from build123d import *

# Parameters (mm, degrees)
BOSS_EXTRUDE1_DEPTH     = 10
BOSS_EXTRUDE2_START     = 2.8
BOSS_EXTRUDE2_DEPTH     = 4.4
BOSS_EXTRUDE3_DEPTH     = 45
CUT_EXTRUDE1_DEPTH      = 103.347447452
CUT_EXTRUDE1_DEPTH_BACK = 103.347447452
CUT_EXTRUDE2_START      = -35
CUT_EXTRUDE2_DEPTH      = 35
SKETCH7_R               = 2.625
CUT_EXTRUDE5_DEPTH      = 43.5


with BuildPart() as part:
    # Sketch1 → Boss-Extrude1 (new body)
    with BuildSketch(Plane(origin=(0, 0, 0), x_dir=(1, 0, 0), z_dir=(0, 1, 0))):
        with BuildLine():
            Line((-40.2, -57.876303889), (-40.2, 0))
            ThreePointArc((-40.2, 0), (-36.256585609, 17.363755354), (-25.2, 31.320919527))
            ThreePointArc((-25.2, 31.320919527), (0, 40.2), (25.2, 31.320919527))
            ThreePointArc((25.2, 31.320919527), (36.256585609, 17.363755354), (40.2, 0))
            Line((40.2, 0), (40.2, -57.876303889))
            ThreePointArc((40.2, -57.876303889), (41.890773052, -60.2417112), (44.676121397, -59.40762496))
            ThreePointArc((44.676121397, -59.40762496), (50.25367708, -51.409776352), (55, -42.892316139))
            Line((55, -42.892316139), (55, 0))
            ThreePointArc((55, 0), (0, 55), (-55, 0))
            Line((-55, 0), (-55, -42.892316139))
            ThreePointArc((-55, -42.892316139), (-50.25367708, -51.409776352), (-44.676121397, -59.40762496))
            ThreePointArc((-44.676121397, -59.40762496), (-41.890773052, -60.2417112), (-40.2, -57.876303889))
        make_face()
    extrude(amount=BOSS_EXTRUDE1_DEPTH)

    # Sketch1<5> → Boss-Extrude2 (add)
    with BuildSketch(Plane(origin=(0, 0, 0), x_dir=(1, 0, 0), z_dir=(0, 1, 0)).offset(BOSS_EXTRUDE2_START)):
        with BuildLine():
            ThreePointArc((-25.2, 31.320919527), (-36.256585609, 17.363755354), (-40.2, 0))
            Line((-40.2, 0), (-40.2, -57.876303889))
            Line((-40.2, -57.876303889), (-29.879111138, -45.576347508))
            ThreePointArc((-29.879111138, -45.576347508), (-26.406147584, -39.560998181), (-25.2, -32.720595315))
            Line((-25.2, -32.720595315), (-25.2, 31.320919527))
        make_face()
        with BuildLine():
            ThreePointArc((40.2, 0), (36.256585609, 17.363755354), (25.2, 31.320919527))
            Line((25.2, 31.320919527), (25.2, -32.720595315))
            ThreePointArc((25.2, -32.720595315), (26.406147584, -39.560998181), (29.879111138, -45.576347508))
            Line((29.879111138, -45.576347508), (40.2, -57.876303889))
            Line((40.2, -57.876303889), (40.2, 0))
        make_face()
    extrude(amount=BOSS_EXTRUDE2_DEPTH)

    # Sketch1<6> → Boss-Extrude3 (add)
    with BuildSketch(Plane(origin=(0, 0, 0), x_dir=(1, 0, 0), z_dir=(0, 1, 0))):
        with BuildLine():
            ThreePointArc((-65, 0), (-62.466921066, -22.021300959), (-55, -42.892316139))
            Line((-55, -42.892316139), (-55, 0))
            ThreePointArc((-55, 0), (0, 55), (55, 0))
            Line((55, 0), (55, -42.892316139))
            ThreePointArc((55, -42.892316139), (62.466921066, -22.021300959), (65, 0))
            ThreePointArc((65, 0), (0, 65), (-65, 0))
        make_face()
    extrude(amount=BOSS_EXTRUDE3_DEPTH)

    # Sketch2 → Cut-Extrude1 (cut, two sides: drawn at the far end of the back side and taken through both)
    with BuildSketch(Plane(origin=(0, 0, 0), x_dir=(0, 0, -1), z_dir=(1, 0, 0)).offset(-CUT_EXTRUDE1_DEPTH_BACK)):
        with BuildLine():
            Line((-42.892316139, 10), (-42.892316139, 45))
            Line((-42.892316139, 45), (17.107683861, 45))
            ThreePointArc((17.107683861, 45), (-17.623426113, 35.61047424), (-42.892316139, 10))
        make_face()
    extrude(amount=CUT_EXTRUDE1_DEPTH + CUT_EXTRUDE1_DEPTH_BACK, mode=Mode.SUBTRACT)

    # Sketch3 → Cut-Extrude2 (cut)
    with BuildSketch(Plane(origin=(0, 45, 0), x_dir=(1, 0, 0), z_dir=(0, 1, 0)).offset(CUT_EXTRUDE2_START)):
        with BuildLine():
            Line((-34.164958741, 55.296976357), (-27.5, 47.631397208))
            ThreePointArc((-27.5, 47.631397208), (-36.087479082, 41.505347288), (-43.347496237, 33.852541558))
            ThreePointArc((-43.347496237, 33.852541558), (-47.000937608, 28.564170983), (-50.012454978, 22.885679957))
            Line((-50.012454978, 22.885679957), (-50.012454978, 41.518120707))
            ThreePointArc((-50.012454978, 41.518120707), (-42.648838916, 49.051774067), (-34.164958741, 55.296976357))
        make_face()
        with BuildLine():
            Line((64.971065648, 1.93923401), (55, 0))
            ThreePointArc((55, 0), (53.988424685, 10.5), (50.990909091, 20.613762153))
            ThreePointArc((50.990909091, 20.613762153), (48.237766513, 26.421920479), (44.825807714, 31.869216538))
            Line((44.825807714, 31.869216538), (60.961974739, 22.552996163))
            ThreePointArc((60.961974739, 22.552996163), (63.804501901, 12.409090909), (64.971065648, 1.93923401))
        make_face()
    extrude(amount=CUT_EXTRUDE2_DEPTH, mode=Mode.SUBTRACT)

    # Sketch7 → Cut-Extrude5 (cut)
    with BuildSketch(Plane(origin=(0, 0, 0), x_dir=(0, 1, 0), z_dir=(0.32556815445715737, 0, 0.9455185755993166))):
        with Locations(Location((5, 0, 0), (0, 0, 270))):
            Circle(SKETCH7_R)
    extrude(amount=-CUT_EXTRUDE5_DEPTH, mode=Mode.SUBTRACT)


solid = part.part
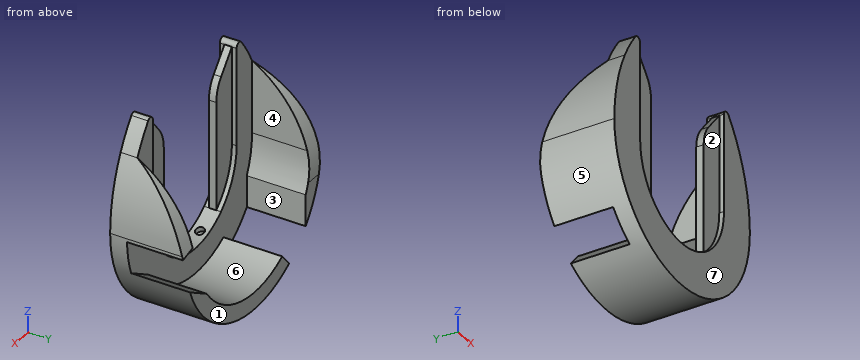
Here's how the part is built. I have some questions about the finished solid (model axes, mm). Face numbers are marked on the shaded views. A direction names the side the tool comes from. Round coordinates to 2 decimals unless told otherwise and drop trailing zeros. Loops run counter-clockwise (first coordinate to the right, second up) from the corner with the lowest first, then second, coordinate; pieces in that order, holes last.
1. We'd pull the mould along X, two halves only. Please class the marked faces 5, 6 and 7: +X half, -X half, draft (parallel to the pull), parting line (faces both ways), or undercut.
Answer list:
face 5: parting line
face 6: undercut
face 7: draft
2. If we section it at B-B on z = 8.5: Write out the boundary of the cut face in (x, y), plus the area to 3 significant figures.
Answer list:
outline: (-64.63, 0) - (-40.2, 0) - (-40.2, 2.8) - (-25.2, 2.8) - (-25.2, 7.2) - (-40.2, 7.2) - (-40.2, 10) - (-55, 10) - (-55, 40.07) - (-64.63, 40.07) - close; (25.2, 2.8) - (40.2, 2.8) - (40.2, 0) - (64.63, 0) - (64.63, 40.07) - (55, 40.07) - (55, 10) - (40.2, 10) - (40.2, 7.2) - (25.2, 7.2) - close
area: 1,200 mm2
3. If we section it at A-A on y = 19.5: Write out the boundary of the cut face in (x, z), plus the area to 3 significant figures.
Answer list:
outline: (-65, 0) arc R65 ccw to (-50.01, -41.52) - (-50.01, -22.89) arc R55 cw to (-55, 0) - (-55, 36.42) - (-57.9, 36.42) arc R96.99 ccw to start; (-34.16, -55.3) arc R65 ccw to (60.96, -22.55) - (44.83, -31.87) arc R55 cw to (-27.5, -47.63) - close; (55, 0) - (64.97, -1.94) arc R65 ccw to (65, 0) arc R96.99 ccw to (57.9, 36.42) - (55, 36.42) - close
area: 1,900 mm2
4. If we section it at C-C on x = 0: Write out the boundary of the cut face in (y, z).
Answer list:
outline: (0, -65) - (45, -65) - (45, -55) - (10, -55) - (10, -40.2) - (0, -40.2) - close
5. Which directions (+Z, -Z, +X, -X, +Y, -Y) give clear straight access to the entire face, cutting with the end or side of a thin tool? Please do the marked faces 1, 2, 3 and 4.
Answer list:
face 1: +Z, -Z, +X, -X, +Y
face 2: +Z, -Y
face 3: +Z, -Z, +Y
face 4: +Z, +Y
6. For P1, Ø4.5, axis at x = -35, z = 9.5, coming from the -Y side; P2, Ø15, axis at y = 30, z = -33.5, coming from the +X side; P3, Ø12, axis at x = 34.5, z = -5, coming from the +Y side; P4, Ø10, axis at x = -39.5, y = 32, coming from the -Z side, each with a flat end and sliding along its axis, tell me the tip position at first contact or that it passes through.
Answer list:
P1: stops at y = 2.8
P2: stops at x = 59.57
P3: stops at y = 10
P4: passes through
7. If we section it at D-D on y = 29: Write out the boundary of the cut face in (x, z).
Answer list:
outline: (-65, 0) arc R65 ccw to (-50.01, -41.52) - (-50.01, -22.89) arc R55 cw to (-55, 0) - (-55, 27.05) - (-61.15, 27.05) arc R96.99 ccw to start; (-34.16, -55.3) arc R65 ccw to (60.96, -22.55) - (44.83, -31.87) arc R55 cw to (-27.5, -47.63) - close; (55, 0) - (64.97, -1.94) arc R65 ccw to (65, 0) arc R96.99 ccw to (61.15, 27.05) - (55, 27.05) - close
8. If I drill on line 1 along Y through (x, z) = (28.5, -39); line 2 along Y through (x, z) = (30, 41.5); line 3 along X through (y, z) = (21, -28.5), over which ranges is the centre line in solid material (lowest first)?
Answer list:
line 1: y = 0 to 10
line 2: y = 2.8 to 7.2
line 3: x = -58.42 to -50.01, 50.66 to 58.42
